from build123d import *

# Parameters (mm, degrees)
SKETCH1_R                                     = 8.89
TRAINGULAR_BASE_SIMPLIFIED_TO_CIRCLE_HE_DEPTH = 4
SKETCH2_R                                     = 5
DRIVE_SHAFT_DEPTH                             = 33.782
SKETCH4_R                                     = 5
SKETCH4_R_2                                   = 4.238
RETAINING_RING_SLOT_DEPTH                     = 1.143
HEX_SLOT_DEPTH                                = 12.7


with BuildPart() as part:
    # Sketch1 → Traingular base (simplified to circle here) (new body)
    with BuildSketch(Plane(origin=(0, 0, 0), x_dir=(1, 0, 0), z_dir=(0, 1, 0))):
        with Locations(Location((0, 0, 0), (0, 0, 270))):
            Circle(SKETCH1_R)
    extrude(amount=TRAINGULAR_BASE_SIMPLIFIED_TO_CIRCLE_HE_DEPTH)

    # Sketch2 → Drive shaft (add)
    with BuildSketch(Plane(origin=(0, 4, 0), x_dir=(1, 0, 0), z_dir=(0, 1, 0))):
        with Locations(Location((0, 0, 0), (0, 0, 270))):
            Circle(SKETCH2_R)
    extrude(amount=DRIVE_SHAFT_DEPTH)

    # Sketch4 → Retaining ring slot (cut)
    with BuildSketch(Plane(origin=(0, 21.272, 0), x_dir=(1, 0, 0), z_dir=(0, 1, 0))):
        with Locations(Location((0, 0, 0), (0, 0, 270))):
            Circle(SKETCH4_R)
        with Locations(Location((0, 0, 0), (0, 0, 270))):
            Circle(SKETCH4_R_2, mode=Mode.SUBTRACT)
    extrude(amount=RETAINING_RING_SLOT_DEPTH, mode=Mode.SUBTRACT)

    # Sketch5 → Hex slot (cut)
    with BuildSketch(Plane(origin=(0, 37.782, 0), x_dir=(1, 0, 0), z_dir=(0, 1, 0))):
        Polygon((3.6449, 0), (1.82245, 3.156575994), (-1.82245, 3.156575994), (-3.6449, 0), (-1.82245, -3.156575994), (1.82245, -3.156575994), align=None)
    extrude(amount=-HEX_SLOT_DEPTH, mode=Mode.SUBTRACT)


solid = part.part
Build history of the part. All positions in model axes, mm. A direction names the side the tool comes from. Round coordinates to 2 decimals unless told otherwise and drop trailing zeros. Order: outer loops, then holes, each group sorted by start corner. A loop starts at its lowest first (then second) coordinate and runs counter-clockwise, first axis right, second up. Notation, with made-up numbers: M 39,-24.5 L 67,-24.5 A7 ccw 67,-14.5 Z; hole C 81,87 d1. An arc over 180 degrees is marked long. Use CSV: the item, a comma, the result in double quotes. Start each with the question number.
(1) Cut at B-B on x = 0. List the corners of the cut face in (y, z) (3 decimals), then the cut area to 3 significant figures.
(2) Cut at A-A on y = 26. List the corners of the cut face in (x, z), then the cut area to 3 significant figures.
(3) Mould opens along X. For faces 1 (the face through (-4.88, 29.99, -1.08)), 2 (the face through (0, 25.082, 0)), 3 (the face through (2, 21.272, -4)), 4 (the face through (0, 32, -3.157)) say: +X half, -X half, draft (parallel to the pull), parting line (faces both ways), or undercut.
(4) Tool access for faces 5 (the face through (-8.68, 1.97, -1.93)), 6 (the face through (1.273, 21.835, 4.042)), 7 (the face through (-2.746, 31.521, 1.556)): list every direction of +Z, -Z, +X, -X, +Y, -Y with a clear straight run to the whole face (end or side of a thin tool).
(5) Flat gauge pins, fed straight in: P1, Ø3, axis at x = -0.5, z = -0.5, coming from the +Y side; P2, Ø1.8, axis at x = -0.5, y = 30.5, coming from the -Z side; P3, Ø1.8, axis at x = -0.5, y = 28.5, coming from the +Z side. Where does each tip first touch, or does it go through?
(6) Drill centre lines: probe 1 along Y at (x, z) = (-3, 7); probe 2 along Z at (x, y) = (1.5, 33); probe 3 along Z at (x, y) = (1.75, 27.5). Where is each one in solid material? Low to high.
(7) Cut at C-C on z = 3.75. List the corners of the cut face in (x, y) (3 decimals).
(8) Cut at D-D on y = 3.5. List the corners of the cut face in (x, z), then the cut area to 3 significant figures.
Findings:
1,outline,"M 0,-8.89 L 4,-8.89 L 4,-5 L 21.272,-5 L 21.272,-4.238 L 22.415,-4.238 L 22.415,-5 L 37.782,-5 L 37.782,-3.157 L 25.082,-3.157 L 25.082,3.157 L 37.782,3.157 L 37.782,5 L 22.415,5 L 22.415,4.238 L 21.272,4.238 L 21.272,5 L 4,5 L 4,8.89 L 0,8.89 Z"
1,area,"327 mm^2"
2,outline,"C 0,0 d10; hole M -3.64,0 L -1.82,-3.16 L 1.82,-3.16 L 3.64,0 L 1.82,3.16 L -1.82,3.16 Z"
2,area,"44.0 mm^2"
3,face 1,"parting line"
3,face 2,"undercut"
3,face 3,"draft"
3,face 4,"undercut"
4,face 5,"+Y, -Y"
4,face 6,"none"
4,face 7,"+Y"
5,P1,"stops at y = 25.08"
5,P2,"stops at z = -5"
5,P3,"stops at z = 5"
6,probe 1,"y = 0 to 4"
6,probe 2,"z = -4.77 to -3.16, 3.16 to 4.77"
6,probe 3,"z = -4.68 to -3.16, 3.16 to 4.68"
7,outline,"M -8.06,0 L 8.06,0 L 8.06,4 L 3.307,4 L 3.307,21.272 L 1.974,21.272 L 1.974,22.415 L 3.307,22.415 L 3.307,37.782 L -3.307,37.782 L -3.307,22.415 L -1.974,22.415 L -1.974,21.272 L -3.307,21.272 L -3.307,4 L -8.06,4 Z"
8,outline,"C 0,0 d17.78"
8,area,"248 mm^2"
